Source: CAD feature listing. Evaluate the final solid. Frame: model axes, mm. A direction names the side the tool comes from. Round coordinates to 2 decimals unless told otherwise and drop trailing zeros. Loops run counter-clockwise (first coordinate to the right, second up) from the corner with the lowest first, then second, coordinate; pieces in that order, holes last. Notation, with made-up numbers: (-5.75, 58) -> (26.25, 58) arc R22 cw to (26.25, 88) -> close; hole circle Ø10 at (80.5, 15). An arc over 180 degrees is marked (long way). Return JSON: item names as keys, results as strings. Group by question number.
Autodesk Inventor part; units mm, degrees
ref_plane "XY Plane" through (0, 0, 0) normal (0, 0, 1) x (1, 0, 0)
sketch "Sketch1" plane through (0, 0, 0) normal (1, 0, 0) x (0, 1, 0)
  line L0 (0, 0) -> (31.5, 0)
  line L1 (31.5, 0) -> (31.5, -14)
  line L2 (31.5, -14) -> (0, -14)
  line L3 (0, -14) -> (0, 0) construction
  line L4 (27, 0) -> (31.5, -12)
  line L5 (0, 0) -> (12, 0)
  line L6 (12, 0) -> (12, -14)
  line L7 (12, -14) -> (0, -14)
  line L8 (0, -14) -> (0, 0) construction
  dimension "d0" = 31.5
  dimension "d1" = 14
  dimension "d2" = 2
  dimension "d3" = 27
  dimension "d4" = 12
revolve "Revolution1" add sketch "Sketch1" angle 360 about axis through (0, 0, -14) along (0, 0, 1) contours L0 L4 L1 L2 L6
fillet "Fillet1" radius 2 1 edges at (0, -27, 0)
shell "Shell1" thickness 1.5875 removed faces 1 at (2.5128, 24.6949, -14)
sketch "Sketch2" plane through (0, 0, 0) normal (0, 0, 1) x (1, 0, 0)
  circle A0 centre (0, 0) radius 15 construction
  circle A1 centre (0, 0) radius 22 construction
  line L0 (0, 0) -> (0, 22) construction
  circle A2 centre (0, 15) radius 2
  circle A3 centre (0, 22) radius 2
  circle A4 centre (-22, 0) radius 2
  circle A5 centre (-15, 0) radius 2
  circle A6 centre (0, -22) radius 2
  circle A7 centre (0, -15) radius 2
  circle A8 centre (22, 0) radius 2
  circle A9 centre (15, 0) radius 2
  dimension "d7" = 30
  dimension "d8" = 44
  dimension "d9" = 4
  dimension "d10" = 4
  dimension "d13" = 360
extrude "Extrusion1" cut sketch "Sketch2" against normal blind 25.4
ref_plane "Work Plane1" through (0, 0, 0) normal (-0.7071, 0.7071, 0) x (0, 0, 1)
sketch "Sketch3" plane through (0, 0, 0) normal (-0.7071, 0.7071, 0) x (0, 0, 1)
  line L0 (-14, 8.6088) -> (-14, -8.6088)
  line L1 (-14, 0) -> (0, 0) construction
  line L2 (-7, -5) -> (-7, 5) construction
  line L3 (-14, 8.6088) -> (-1.5875, 8.6088)
  line L4 (-3, -5) -> (-3, 5)
  line L5 (-11, 5) -> (-11, -5)
  arc A0 (-11, -5) -> (-3, -5) centre (-7, -5) ccw
  arc A1 (-3, 5) -> (-11, 5) centre (-7, 5) ccw
  line L6 (-7, 0) -> (3, 0) construction
  point P0 (-5.2748, 8.6088)
  point P1 (-8.7252, 8.6088)
  dimension "d18" = 5
  dimension "d19" = 90
  dimension "d20" = 8
extrude "Extrusion2" cut sketch "Sketch3" against normal blind 50.8 contours L3 A1 L4 A0 L5
properties part number "Base" material "Stainless Steel"
(1) Ray query, line 1 (X direction, y = -11, z = -6.75); line 2 (Y direction, x = -7, z = -11.5); line 3 (Y direction, x = 2, z = -6). Return the intervals inside material, ascending.
(2) Pin query (flat end, axial travel): pin 1 (4 mm diameter, centred on x = 17, y = -18.5, fed in from -Z); pin 2 (2 mm diameter, centred on y = -12, z = -10.5, fed in from +X); pin 3 (6.5 mm diameter, centred on x = 19.5, y = -22.5, fed in from +Z). Return the tip coordinate at first contact, or that it passes through.
(3) Mould query, pull axis X, two halves, no side actions, for faces 5 (the face through (0.34, -12.683, -8.45)), 6 (the face through (11, 5.3, 0)), 7 (the face through (13.306, -26.034, -7.029)), 8 (the face through (-24.61, 12.8, -1.97)). Classes: released by +X, released by -X, zero draft, split by the parting line, or undercut.
(4) Cut plane C-C (x = 21). Count the separate pieces of the cut face and the enclosed holes in it, and give its area (3 significant figures).
(5) Cut plane B-B (z = -4). Return loops of the section in (x, y) (1 decimal).
(6) Set-up query: faces 1 (the face through (25.486, -13.311, -7.024)), 2 (the face through (0.923, 20.226, -0.783)), 3 (the face through (12.43, -2.38, -3.6)), 4 (the face through (9.7, -9.515, -12.018)). Return all of +Z, -Z, +X, -X, +Y, -Y with unobstructed straight access to the full face (end or side cutting, diameter ignored); none if empty.
Answers follow:
{
 "1": {"line 1": "-27.41 to -25.57, -7.98 to -4.8, 25.57 to 27.41", "line 2": "-30.52 to -28.78, -11.65 to -9.75, 9.75 to 11.65, 28.78 to 30.52", "line 3": "-29.18 to -27.48, 11.83 to 13.44, 27.48 to 29.18"},
 "2": {"pin 1": "z = -3", "pin 2": "x = 29.09", "pin 3": "z = -0.22"},
 "3": {"face 5": "undercut", "face 6": "zero draft", "face 7": "released by +X", "face 8": "split by the parting line"},
 "4": {"separate pieces": "3", "enclosed holes": "0", "area": "89.8 mm^2"},
 "5": {"outline": "(-13.5, -1.3) arc R13.6 ccw to (-1.3, -13.5) arc R2 cw to (1.3, -13.5) arc R13.6 ccw to (2.5, -13.3) -> (1.1, -11.9) arc R12 cw (long way) to (11.9, -1.1) -> (13.3, -2.5) arc R13.6 ccw to (13.5, -1.3) arc R2 cw to (13.5, 1.3) arc R13.6 ccw to (1.3, 13.5) arc R2 cw to (-1.3, 13.5) arc R13.6 ccw to (-13.5, 1.3) arc R2 cw to start; (12.8, -23.6) arc R26.8 cw (long way) to (23.6, -12.8) -> (24.8, -14) arc R28.5 ccw (long way) to (14, -24.8) -> close"},
 "6": {"face 1": "-Y", "face 2": "+Z, -Z", "face 3": "none", "face 4": "-Z"}
}
